Read the model definition and answer for the solid it produces. Units are mm, in the model's axes. Face numbers are marked on the shaded views. Give positions to 0.01 mm unless a question says otherwise; leave off trailing zeros. Order: outer loops, then holes, each group sorted by start corner. A loop starts at its lowest first (then second) coordinate and runs counter-clockwise, first axis right, second up. Notation, with made-up numbers: (54.25, 73.5) -> (100.25, 73.5) arc R31 ccw to (100.25, 109.5) -> close; hole circle Ø7 at (68.25, -15.75). An arc over 180 degrees is marked (long way). Answer as CSV lines item,"result". Start each with the question number.
1) Flat-ended cylindrical pins translate along their axes: pin 1 Ø2 at (x, y) = (7.5, 90.5) entering from +Z; pin 2 Ø3.5 at (x, y) = (-45.5, 89) entering from +Z; pin 3 Ø3 at (x, z) = (47.5, 3.5) entering from +Y; pin 4 Ø10 at (x, y) = (-32.5, 39.5) entering from -Z. Find the tip coordinate at first contact, or state that the pin passes through.
2) Straight lines are drawn through the part: L1, parallel to Y at x = 0, z = 0.6; L2, parallel to Y at x = -24, z = 0.55; L3, parallel to X at y = 82.5, z = 0.55. For each, find the intervals that lie inside material, in ascending order. Write a range as from..to.
3) Find section B-B (y = 16.5). Determine the outline of the cut face in (x, z), and give its area (3 significant figures).
4) Find section D-D (z = 1.2). State how many separate pieces and enclosed holes the cut face has, and give its area (3 significant figures).
5) Find section C-C (y = 82). Determine the outline of the cut face in (x, z), and give its area (3 significant figures).
6) Find section A-A (x = -14). Determine the outline of the cut face in (y, z), and give its area (3 significant figures).
7) The mould has two halves that part along Y. Classify the marked faces 1 and 2: +Y half, -Y half, draft (parallel to the pull), parting line (faces both ways), or undercut.
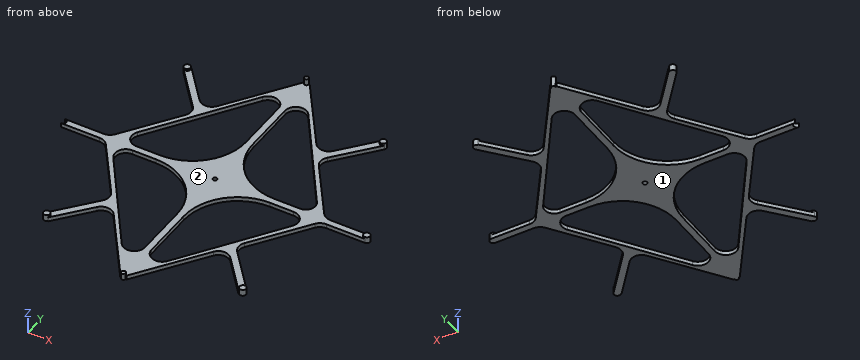
```python
from build123d import *

# Parameters (mm, degrees)
F0_R     = 1
F1_DEPTH = 2
F2_DEPTH = 3
F3_DEPTH = 5


with BuildPart() as f1:
    # F0 (on Top) → F1 (new body)
    with BuildSketch(Plane.XY):
        with BuildLine():
            Line((1, -35.1), (1.5, -35.1))
            Line((1.5, -35.1), (23.193478, -4.3713))
            ThreePointArc((23.193478, -4.3713), (26.906428, -2.344127), (30.781196, -4.041655))
            Line((30.781196, -4.041655), (44.164128, -19.880392))
            Line((44.164128, -19.880392), (44.35536, -19.718811))
            ThreePointArc((44.35536, -19.718811), (44.533011, -17.604942), (46.64688, -17.782593))
            Line((46.64688, -17.782593), (31.206023, 0.491704))
            ThreePointArc((31.206023, 0.491704), (30.029934, 3.501716), (30.940547, 6.602383))
            Line((30.940547, 6.602383), (48.505924, 31.483649))
            ThreePointArc((48.505924, 31.483649), (50.290408, 33.039496), (52.590599, 33.6))
            Line((52.590599, 33.6), (70.5, 33.6))
            ThreePointArc((70.5, 33.6), (69, 35.1), (70.5, 36.6))
            Line((70.5, 36.6), (52.590599, 36.6))
            ThreePointArc((52.590599, 36.6), (50.290408, 37.160504), (48.505924, 38.716351))
            Line((48.505924, 38.716351), (30.940547, 63.597617))
            ThreePointArc((30.940547, 63.597617), (30.029934, 66.698284), (31.206023, 69.708296))
            Line((31.206023, 69.708296), (46.64688, 87.982593))
            ThreePointArc((46.64688, 87.982593), (44.533011, 87.804942), (44.35536, 89.918811))
            Line((44.35536, 89.918811), (44.164128, 90.080392))
            Line((44.164128, 90.080392), (30.948157, 74.439253))
            ThreePointArc((30.948157, 74.439253), (26.91194, 72.670995), (23.044283, 74.782634))
            Line((23.044283, 74.782634), (1.5, 105.3))
            Line((1.5, 105.3), (1, 105.3))
            ThreePointArc((1, 105.3), (0, 104.3), (-1, 105.3))
            Line((-1, 105.3), (-1.5, 105.3))
            Line((-1.5, 105.3), (-23.044283, 74.782634))
            ThreePointArc((-23.044283, 74.782634), (-26.91194, 72.670995), (-30.948157, 74.439253))
            Line((-30.948157, 74.439253), (-44.164128, 90.080392))
            Line((-44.164128, 90.080392), (-44.35536, 89.918811))
            ThreePointArc((-44.35536, 89.918811), (-44.092461, 89.466144), (-44.00112, 88.950702))
            ThreePointArc((-44.00112, 88.950702), (-44.985678, 87.542043), (-46.64688, 87.982593))
            Line((-46.64688, 87.982593), (-31.206023, 69.708296))
            ThreePointArc((-31.206023, 69.708296), (-30.029934, 66.698284), (-30.940547, 63.597617))
            Line((-30.940547, 63.597617), (-48.505924, 38.716351))
            ThreePointArc((-48.505924, 38.716351), (-50.290408, 37.160504), (-52.590599, 36.6))
            Line((-52.590599, 36.6), (-70.5, 36.6))
            ThreePointArc((-70.5, 36.6), (-69.43934, 36.16066), (-69, 35.1))
            ThreePointArc((-69, 35.1), (-69.43934, 34.03934), (-70.5, 33.6))
            Line((-70.5, 33.6), (-52.590599, 33.6))
            ThreePointArc((-52.590599, 33.6), (-50.290408, 33.039496), (-48.505924, 31.483649))
            Line((-48.505924, 31.483649), (-30.940547, 6.602383))
            ThreePointArc((-30.940547, 6.602383), (-30.029934, 3.501716), (-31.206023, 0.491704))
            Line((-31.206023, 0.491704), (-46.64688, -17.782593))
            ThreePointArc((-46.64688, -17.782593), (-44.985678, -17.342043), (-44.00112, -18.750702))
            ThreePointArc((-44.00112, -18.750702), (-44.092461, -19.266144), (-44.35536, -19.718811))
            Line((-44.35536, -19.718811), (-44.164128, -19.880392))
            Line((-44.164128, -19.880392), (-30.948157, -4.239253))
            ThreePointArc((-30.948157, -4.239253), (-26.91194, -2.470995), (-23.044283, -4.582634))
            Line((-23.044283, -4.582634), (-1.5, -35.1))
            Line((-1.5, -35.1), (-1, -35.1))
            ThreePointArc((-1, -35.1), (0, -34.1), (1, -35.1))
        make_face()
        with BuildLine():
            ThreePointArc((-26.5, 33.6), (-8.82233, 26.27767), (-1.5, 8.6))
            Line((-1.5, 8.6), (-1.5, -16.098123))
            ThreePointArc((-1.5, -16.098123), (-5.008784, -20.870573), (-10.61051, -18.944823))
            Line((-10.61051, -18.944823), (-41.565831, 25.753299))
            ThreePointArc((-41.565831, 25.753299), (-41.884401, 30.920183), (-37.455321, 33.6))
            Line((-37.455321, 33.6), (-26.5, 33.6))
        make_face(mode=Mode.SUBTRACT)
        with BuildLine():
            Line((1.5, -16.098123), (1.5, 8.6))
            ThreePointArc((1.5, 8.6), (8.82233, 26.27767), (26.5, 33.6))
            Line((26.5, 33.6), (37.455321, 33.6))
            ThreePointArc((37.455321, 33.6), (41.884401, 30.920183), (41.565831, 25.753299))
            Line((41.565831, 25.753299), (10.61051, -18.944823))
            ThreePointArc((10.61051, -18.944823), (5.008784, -20.870573), (1.5, -16.098123))
        make_face(mode=Mode.SUBTRACT)
        with BuildLine():
            Line((-1.5, 86.298123), (-1.5, 61.6))
            ThreePointArc((-1.5, 61.6), (-8.82233, 43.92233), (-26.5, 36.6))
            Line((-26.5, 36.6), (-37.455321, 36.6))
            ThreePointArc((-37.455321, 36.6), (-41.884401, 39.279817), (-41.565831, 44.446701))
            Line((-41.565831, 44.446701), (-10.61051, 89.144823))
            ThreePointArc((-10.61051, 89.144823), (-5.008784, 91.070573), (-1.5, 86.298123))
        make_face(mode=Mode.SUBTRACT)
        with Locations((0, 35.1)):
            Circle(F0_R, mode=Mode.SUBTRACT)
        with BuildLine():
            ThreePointArc((26.5, 36.6), (8.82233, 43.92233), (1.5, 61.6))
            Line((1.5, 61.6), (1.5, 86.298123))
            ThreePointArc((1.5, 86.298123), (5.008784, 91.070573), (10.61051, 89.144823))
            Line((10.61051, 89.144823), (42.190267, 43.545043))
            ThreePointArc((42.190267, 43.545043), (42.47223, 38.971882), (38.552092, 36.6))
            Line((38.552092, 36.6), (26.5, 36.6))
        make_face(mode=Mode.SUBTRACT)
    extrude(amount=F1_DEPTH)

    # F0 (on Top) → F2 (join)
    with BuildSketch(Plane.XY):
        with BuildLine():
            ThreePointArc((-44.35536, 89.918811), (-46.469229, 90.096461), (-46.64688, 87.982593))
            ThreePointArc((-46.64688, 87.982593), (-44.985678, 87.542043), (-44.00112, 88.950702))
            ThreePointArc((-44.00112, 88.950702), (-44.092461, 89.466144), (-44.35536, 89.918811))
        make_face()
        with BuildLine():
            ThreePointArc((-1, 105.3), (0, 104.3), (1, 105.3))
            ThreePointArc((1, 105.3), (0, 106.3), (-1, 105.3))
        make_face()
        with BuildLine():
            ThreePointArc((44.35536, 89.918811), (44.533011, 87.804942), (46.64688, 87.982593))
            ThreePointArc((46.64688, 87.982593), (46.909779, 88.43526), (47.00112, 88.950702))
            ThreePointArc((47.00112, 88.950702), (46.016562, 90.359361), (44.35536, 89.918811))
        make_face()
        with BuildLine():
            ThreePointArc((70.5, 36.6), (69, 35.1), (70.5, 33.6))
            ThreePointArc((70.5, 33.6), (71.56066, 34.03934), (72, 35.1))
            ThreePointArc((72, 35.1), (71.56066, 36.16066), (70.5, 36.6))
        make_face()
        with BuildLine():
            ThreePointArc((46.64688, -17.782593), (44.533011, -17.604942), (44.35536, -19.718811))
            ThreePointArc((44.35536, -19.718811), (46.016562, -20.159361), (47.00112, -18.750702))
            ThreePointArc((47.00112, -18.750702), (46.909779, -18.23526), (46.64688, -17.782593))
        make_face()
        with BuildLine():
            ThreePointArc((-1, -35.1), (0, -36.1), (1, -35.1))
            ThreePointArc((1, -35.1), (0, -34.1), (-1, -35.1))
        make_face()
        with BuildLine():
            ThreePointArc((-46.64688, -17.782593), (-46.469229, -19.896461), (-44.35536, -19.718811))
            ThreePointArc((-44.35536, -19.718811), (-44.092461, -19.266144), (-44.00112, -18.750702))
            ThreePointArc((-44.00112, -18.750702), (-44.985678, -17.342043), (-46.64688, -17.782593))
        make_face()
    extrude(amount=F2_DEPTH)

    # F0 (on Top) → F3 (join)
    with BuildSketch(Plane.XY):
        with BuildLine():
            ThreePointArc((-1, 105.3), (0, 104.3), (1, 105.3))
            ThreePointArc((1, 105.3), (0, 106.3), (-1, 105.3))
        make_face()
    extrude(amount=F3_DEPTH)


solid = f1.part
```
Findings below:
1,pin 1,"z = 2"
1,pin 2,"z = 3"
1,pin 3,"y = 90.33"
1,pin 4,"z = 0"
2,L1,"-36.1..34.1, 36.1..106.3"
2,L2,"-3.57..0.39, 33.47..36.73, 69.81..73.77"
2,L3,"-42.01..-37.76, -17.6..-15.21, -1.5..1.5, 15.21..17.6, 37.76..42.01"
3,outline,"(-37.93, 0) -> (-35.16, 0) -> (-35.16, 2) -> (-37.93, 2) -> close; (-2.78, 0) -> (2.78, 0) -> (2.78, 2) -> (-2.78, 2) -> close; (35.16, 0) -> (37.93, 0) -> (37.93, 2) -> (35.16, 2) -> close"
3,area,"22.2 mm²"
4,separate pieces,"1"
4,enclosed holes,"5"
4,area,"2,750 mm²"
5,outline,"(-41.59, 0) -> (-37.34, 0) -> (-37.34, 2) -> (-41.59, 2) -> close; (-17.95, 0) -> (-15.56, 0) -> (-15.56, 2) -> (-17.95, 2) -> close; (-1.5, 0) -> (1.5, 0) -> (1.5, 2) -> (-1.5, 2) -> close; (15.56, 0) -> (17.95, 0) -> (17.95, 2) -> (15.56, 2) -> close; (37.34, 0) -> (41.59, 0) -> (41.59, 2) -> (37.34, 2) -> close"
5,area,"32.6 mm²"
6,outline,"(-17.39, 0) -> (-14.05, 0) -> (-14.05, 2) -> (-17.39, 2) -> close; (30.25, 0) -> (39.95, 0) -> (39.95, 2) -> (30.25, 2) -> close; (84.25, 0) -> (87.59, 0) -> (87.59, 2) -> (84.25, 2) -> close"
6,area,"32.8 mm²"
7,face 1,"draft"
7,face 2,"undercut"
